Geometry: final body of the model. Coordinates: model frame, mm. Face numbers are marked on the shaded views. A direction names the side the tool comes from. Round coordinates to 2 decimals unless told otherwise and drop trailing zeros. Loops run counter-clockwise (first coordinate to the right, second up) from the corner with the lowest first, then second, coordinate; pieces in that order, holes last. Notation, with made-up numbers: (-15.75, 61.25) -> (7.25, 61.25) arc R21 ccw to (7.25, 91.25) -> close; hole circle Ø6 at (80.25, 4). An arc over 180 degrees is marked (long way). Answer in a Markdown table with one row per item.
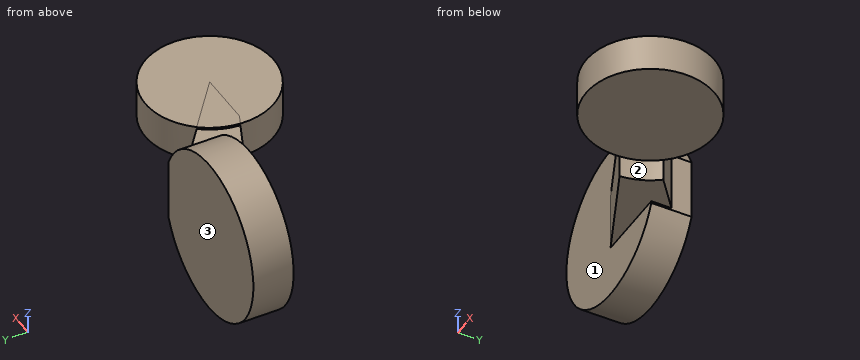
```python
from build123d import *

# Parameters (mm, degrees)
SKETCH1_R           = 200
BOSS_EXTRUDE1_DEPTH = 100
CUT_EXTRUDE2_DEPTH  = 100
BOSS_EXTRUDE2_DEPTH = 75.993421
BOSS_EXTRUDE3_DEPTH = 75.993421
SKETCH9_R           = 159.375
BOSS_EXTRUDE4_DEPTH = 151.986842
CUT_EXTRUDE3_START  = -60
SKETCH11_R          = 159.375
CUT_EXTRUDE3_DEPTH  = 60
CUT_EXTRUDE4_DEPTH  = 5
CUT_EXTRUDE5_DEPTH  = 5


with BuildPart() as part:
    # Sketch1 → Boss-Extrude1 (new body)
    with BuildSketch(Plane(origin=(0, 0, 0), x_dir=(1, 0, 0), z_dir=(0, 1, 0))):
        with Locations(Location((0, 0, 0), (0, 0, 270))):
            Circle(SKETCH1_R)
    extrude(amount=BOSS_EXTRUDE1_DEPTH)

    # Sketch2 → Cut-Extrude2 (cut)
    with BuildSketch(Plane(origin=(0, 100, 0), x_dir=(1, 0, 0), z_dir=(0, 1, 0))):
        Polygon((185, 0), (185, 120.642549135), (200, 120.642549135), (200, 0), (200, -137.849885779), (185, -137.849885779), align=None)
    extrude(amount=-CUT_EXTRUDE2_DEPTH, mode=Mode.SUBTRACT)

    # Sketch4 → Boss-Extrude2 (add)
    with BuildSketch(Plane.XY):
        Polygon((185, 50), (185, 0), (0, 0), (251.924557131, -112.966443103), (387.075695624, -112.966443103), align=None)
    extrude(amount=-BOSS_EXTRUDE2_DEPTH)

    # Sketch7 → Boss-Extrude3 (add)
    with BuildSketch(Plane.XY):
        Polygon((0, 0), (185, 0), (185, 50), (387.075695624, -112.966443103), (251.924557131, -112.966443103), align=None)
    extrude(amount=BOSS_EXTRUDE3_DEPTH)

    # Sketch9 → Boss-Extrude4 (add)
    with BuildSketch(Plane.XY.offset(75.993420768)):
        with Locations((387.075695624, -112.966443103)):
            Circle(SKETCH9_R)
    extrude(amount=-BOSS_EXTRUDE4_DEPTH)

    # Sketch11 → Cut-Extrude3 (cut)
    with BuildSketch(Plane(origin=(0, 0, -75.993420768), x_dir=(-1, 0, 0), z_dir=(0, 0, -1)).offset(CUT_EXTRUDE3_START)):
        with Locations((-387.075695624, -112.966443103)):
            Circle(SKETCH11_R)
    extrude(amount=CUT_EXTRUDE3_DEPTH, mode=Mode.SUBTRACT)


with BuildPart() as cut_extrude3_kept_piece:
    # of the separate pieces the step leaves, the one the design keeps (cut_extrude3_pieces_kept)
    add(part.part.solids().sort_by_distance((185, 0, -75.993420884))[0])

    # Sketch12 → Cut-Extrude4 (cut)
    with BuildSketch(Plane.XY.offset(75.993420768)):
        with BuildLine():
            Line((185, 0), (0, 0))
            Line((0, 0), (228.060355378, -102.265406172))
            ThreePointArc((228.060355378, -102.265406172), (238.589276077, -54.846272892), (262.770904395, -12.719307371))
            Line((262.770904395, -12.719307371), (185, 50))
            Line((185, 50), (185, 0))
        make_face()
    extrude(amount=-CUT_EXTRUDE4_DEPTH, mode=Mode.SUBTRACT)

    # Sketch14 → Cut-Extrude5 (cut)
    with BuildSketch(Plane(origin=(0, 0, -75.993420768), x_dir=(-1, 0, 0), z_dir=(0, 0, -1))):
        with BuildLine():
            Line((-228.060355378, -102.265406172), (0, 0))
            Line((0, 0), (-185, 0))
            Line((-185, 0), (-185, 50))
            Line((-185, 50), (-263.016769179, -12.917588066))
            ThreePointArc((-263.016769179, -12.917588066), (-238.655621962, -54.898617596), (-228.060355378, -102.265406172))
        make_face()
    extrude(amount=-CUT_EXTRUDE5_DEPTH, mode=Mode.SUBTRACT)


solid = cut_extrude3_kept_piece.part
```
Item 1: Cut plane C-C (y = -201.5). Output: boundary loops of the cut face in (x, z), then the cut area to 3 significant figures.
Answer:
| item | result |
|---|---|
| outline | (254.55, -15.99) -> (519.6, -15.99) -> (519.6, 75.99) -> (254.55, 75.99) -> close |
| area | 24,400 mm² |
Item 2: Cut plane D-D (x = 357.5). Output: boundary loops of the cut face in (y, z).
Answer:
| item | result |
|---|---|
| outline | (-269.57, -15.99) -> (43.64, -15.99) -> (43.64, 75.99) -> (-269.57, 75.99) -> close |
Item 3: Line query: probe 1 along Z at (x, y) = (390, 0); probe 2 along Y at (x, z) = (-21, 90); probe 3 along X at (y, z) = (58, -24.5). Output: solid intervals per line, ascending. Write a range as [from, to].
Answer:
| item | result |
|---|---|
| probe 1 | z = [-15.99, 75.99] |
| probe 2 | y = [0, 100] |
| probe 3 | x = [-198.49, 185] |
Item 4: Pin query (flat end, axial travel): pin 1 Ø12 at (x, z) = (145, 140.5) entering from -Y; pin 2 Ø2 at (y, z) = (-44, -5.5) entering from -X; pin 3 Ø2 at (x, y) = (166.5, -20) entering from -Z. Return the tip coordinate at first contact, or that it passes through.
Answer:
| item | result |
|---|---|
| pin 1 | stops at y = 0 |
| pin 2 | stops at x = 95.89 |
| pin 3 | stops at z = -70.99 |
Item 5: Reachability of the marked faces 1, 2 and 3 from +Z, -Z, +X, -X, +Y, -Y: full face, straight path, thin tool, end or side. Return the list, or none.
Answer:
| item | result |
|---|---|
| face 1 | -X, -Y |
| face 2 | -Z, +X, -Y |
| face 3 | +Z, -Z, +X, -X, +Y |
Item 6: Cut plane A-A (z = 0). Output: boundary loops of the cut face in (x, y) (3 decimals).
Answer:
| item | result |
|---|---|
| outline | (-200, 0) -> (0, 0) -> (228.06, -102.265) arc R159.375 ccw (long way) to (263.017, -12.918) -> (185, 50) -> (185, 100) -> (-200, 100) -> close |
Item 7: Cut plane B-B (x = 17). Output: boundary loops of the cut face in (y, z).
Answer:
| item | result |
|---|---|
| outline | (-7.62, -70.99) -> (0, -70.99) -> (0, -199.28) -> (100, -199.28) -> (100, 199.28) -> (0, 199.28) -> (0, 70.99) -> (-7.62, 70.99) -> close |
